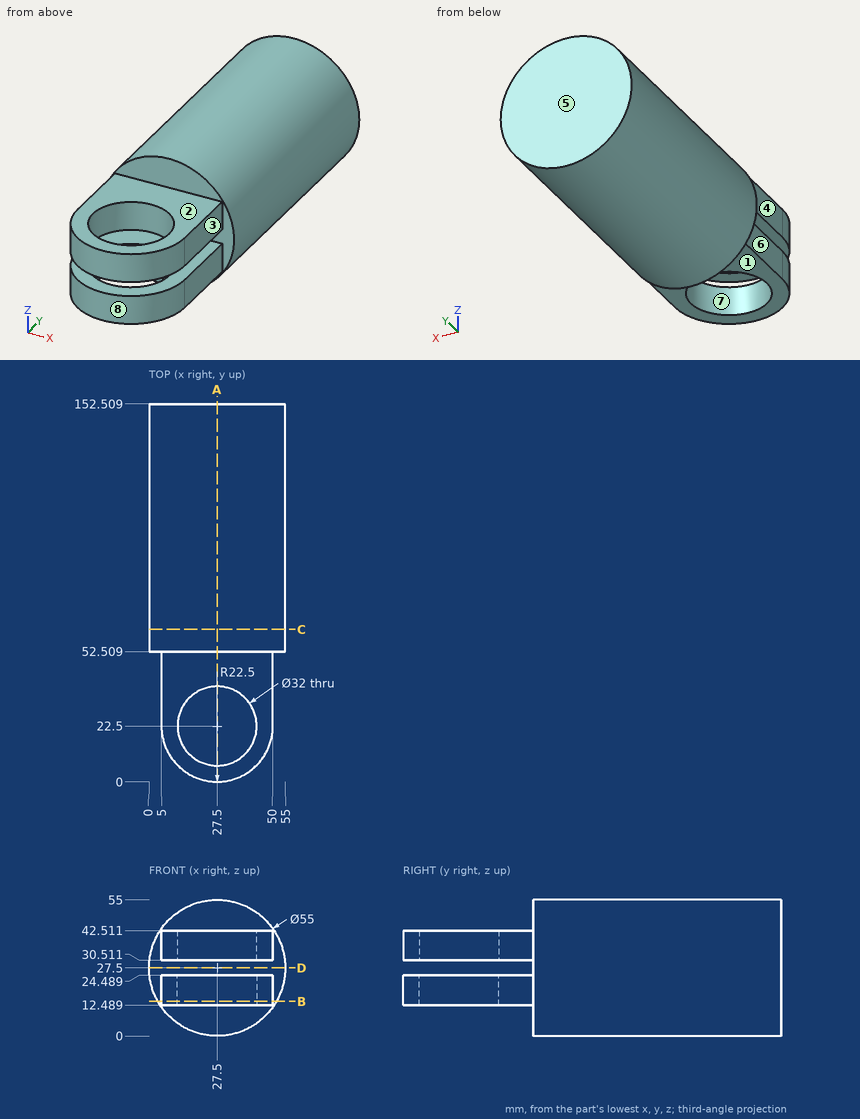
Part print with two shaded views. Sizes in mm from the minimum x, y, z corner. A direction names the side the tool comes from. Round coordinates to 2 decimals unless told otherwise and drop trailing zeros. Order: outer loops, then holes, each group sorted by start corner. A loop starts at its lowest first (then second) coordinate and runs counter-clockwise, first axis right, second up.
(1) Pin check, flat tips, straight feed: pin 1 (22.5 mm diameter, centred on x = 31.5, y = 33, fed in from -Z); pin 2 (3 mm diameter, centred on y = 105, z = 32, fed in from -X); pin 3 (19 mm diameter, centred on x = 27.5, y = 22.5, fed in from -Z); pin 4 (8 mm diameter, centred on y = 121.5, z = 30.5, fed in from +X). Stop position of each tip, or through.
(2) Pull direction X, two halves, no side cores. Call the marked faces 5, 6, 7 and 8: released by +X, released by -X, zero draft, split by the parting line, or undercut.
(3) Band-saw the part on D-D (z = 27.5). List the corners of the cut face in (x, y).
(4) Band-saw the part on B-B (z = 14). List the corners of the cut face in (x, y), then the cut area to 3 significant figures.
(5) Drill centre lines: line 1 (Z direction, x = 30, y = 45); line 2 (Y direction, x = 27, z = 16); line 3 (Z direction, x = 28, y = 87.5). Where is each one in solid material? Low to high.
(6) Band-saw the part on A-A (x = 27.5). List the corners of the cut face in (y, z).
(7) Band-saw the part on C-C (y = 61.5). List the corners of the cut face in (x, z), then the cut area to 3 significant figures.
(8) 3-axis set-ups, long thin cutter, end or side, ignore diameter. For the marked faces 1, 2, 3 and 4: which of +Z, -Z, +X, -X, +Y, -Y reach the whole face in a straight line?
Verdict:
1. pin 1: stops at z = 12.49
1. pin 2: stops at x = 0.16
1. pin 3: passes through
1. pin 4: stops at x = 55
2. face 5: zero draft
2. face 6: released by -X
2. face 7: undercut
2. face 8: split by the parting line
3. outline: (0, 52.51) - (55, 52.51) - (55, 152.51) - (0, 152.51) - close
4. outline: (3.54, 52.51) - (5, 52.51) - (5, 22.51) arc R22.5 ccw to (50, 22.51) - (50, 52.51) - (51.46, 52.51) - (51.46, 152.51) - (3.54, 152.51) - close; hole circle Ø32 at (27.5, 22.5)
4. area: 6,130 mm2
5. line 1: z = 12.49 to 24.49, 30.51 to 42.51
5. line 2: y = 0.01 to 6.51, 38.49 to 152.51
5. line 3: z = 0 to 55
6. outline: (0, 12.49) - (6.5, 12.49) - (6.5, 24.49) - (0, 24.49) - close; (0, 30.51) - (6.5, 30.51) - (6.5, 42.51) - (0, 42.51) - close; (38.5, 12.49) - (52.51, 12.49) - (52.51, 0) - (152.51, 0) - (152.51, 55) - (52.51, 55) - (52.51, 42.51) - (38.5, 42.51) - (38.5, 30.51) - (52.51, 30.51) - (52.51, 24.49) - (38.5, 24.49) - close
7. outline: circle Ø55 at (27.5, 27.5)
7. area: 2,380 mm2
8. face 1: -Z, +X, -X, -Y
8. face 2: +Z, +X, -X, -Y
8. face 3: +Z, -Z, +X, -Y
8. face 4: +Z, -Z, -X, -Y
